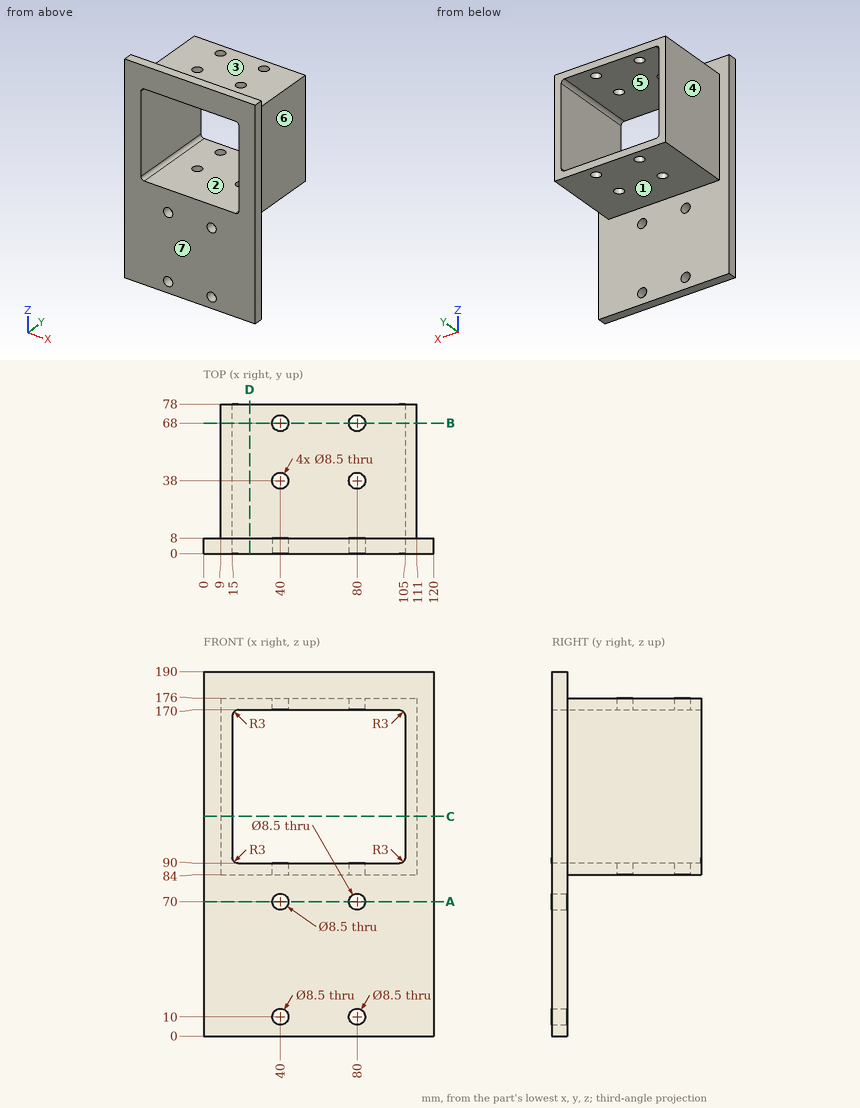
Geometry: see drawing. Coordinates: mm, zero at the bounding-box minimum. A direction names the side the tool comes from. Round coordinates to 2 decimals unless told otherwise and drop trailing zeros. Order: outer loops, then holes, each group sorted by start corner. A loop starts at its lowest first (then second) coordinate and runs counter-clockwise, first axis right, second up. Notation, with made-up numbers: (83.25, 46) - (129.25, 46) arc R17 ccw to (129.25, 65) - close; hole circle Ø6 at (51, 8). An arc over 180 degrees is marked (long way). One line per question, with ' | ' between items. Start each with the question number.
1) Pull-direction query (X, two-part tool) for the marked faces 5, 6 and 7; classes: +X half, -X half, draft (parallel to the pull), parting line (faces both ways), or undercut.
2) Contact query for flat-ended pins moving along their axis: P1, Ø7, axis at x = 40, z = 70, coming from the -Y side; P2, Ø4, axis at x = 98.5, y = 11, coming from the -Z side; P3, Ø11, axis at x = 40, y = 68, coming from the +Z side; P4, Ø6, axis at y = 57, z = 131, coming from the -X side. Output: stop coordinate, or through.
3) Cut plane D-D, the plane x = 24. Return the cut outline in (y, z), then the cut area to 3 significant figures.
4) Ray query, probe 1 along Y at (x, z) = (80, 88); probe 2 along X at (y, z) = (18, 113); probe 3 along Z at (x, y) = (37.5, 58). Return the intervals inside material, ascending.
5) Cut plane C-C, the plane z = 114.5. Return the cut outline in (x, y), then the cut area to 3 significant figures.
6) Cut plane A-A, the plane z = 70. Return the cut outline in (x, y), then the cut area to 3 significant figures.
7) Set-up query: the marked faces 1, 2, 3 and 4. Return all of +Z, -Z, +X, -X, +Y, -Y with unobstructed straight access to the full face (end or side cutting, diameter ignored); none if empty.
8) Cut plane B-B, the plane y = 68. Return the cut outline in (x, z), then the cut area to 3 significant figures.
Worked out:
1) face 5: undercut | face 6: +X half | face 7: draft
2) P1: passes through | P2: stops at z = 84 | P3: stops at z = 176 | P4: stops at x = 9
3) outline: (0, 0) - (8, 0) - (8, 84) - (78, 84) - (78, 90) - (0, 90) - close; (0, 170) - (78, 170) - (78, 176) - (8, 176) - (8, 190) - (0, 190) - close | area: 1,720 mm^2
4) probe 1: y = 0 to 33.75, 42.25 to 63.75, 72.25 to 78 | probe 2: x = 9 to 15, 105 to 111 | probe 3: z = 84 to 90, 170 to 176
5) outline: (0, 0) - (15, 0) - (15, 78) - (9, 78) - (9, 8) - (0, 8) - close; (105, 0) - (120, 0) - (120, 8) - (111, 8) - (111, 78) - (105, 78) - close | area: 1,080 mm^2
6) outline: (0, 0) - (35.75, 0) - (35.75, 8) - (0, 8) - close; (44.25, 0) - (75.75, 0) - (75.75, 8) - (44.25, 8) - close; (84.25, 0) - (120, 0) - (120, 8) - (84.25, 8) - close | area: 824 mm^2
7) face 1: -Z, +X, -X, +Y | face 2: +Y, -Y | face 3: +Z, +X, -X, +Y | face 4: +Z, -Z, -X, +Y
8) outline: (9, 84) - (35.75, 84) - (35.75, 90) - (18, 90) arc R3 cw to (15, 93) - (15, 167) arc R3 cw to (18, 170) - (35.75, 170) - (35.75, 176) - (9, 176) - close; (44.25, 84) - (75.75, 84) - (75.75, 90) - (44.25, 90) - close; (44.25, 170) - (75.75, 170) - (75.75, 176) - (44.25, 176) - close; (84.25, 84) - (111, 84) - (111, 176) - (84.25, 176) - (84.25, 170) - (102, 170) arc R3 cw to (105, 167) - (105, 93) arc R3 cw to (102, 90) - (84.25, 90) - close | area: 1,990 mm^2
